Check sheet for the modelled part. Datum: model origin and axes. Units: mm. A direction names the side the tool comes from. Round coordinates to 2 decimals unless told otherwise and drop trailing zeros. Loops run counter-clockwise (first coordinate to the right, second up) from the corner with the lowest first, then second, coordinate; pieces in that order, holes last. Notation, with made-up numbers: (-21, 63.5) - (33, 63.5) arc R12 cw to (33, 86.5) - close; hole circle Ø8 at (-31.75, 0.25). An arc over 180 degrees is marked (long way). Put each result on its own line as item: value. Start each with the question number.
Item 1: Material ranges on line 1 along X through (y, z) = (-19.5, 0.5); line 2 along X through (y, z) = (-29.5, 0.5); line 3 along Y through (x, z) = (125.5, 4.5), recorded low to high.
Item 2: Gauge pin test, flat ends, axial feed: pin 1 Ø1.9 at (y, z) = (-72, 2) entering from +X; pin 2 Ø3 at (y, z) = (-93, 3) entering from -X; pin 3 Ø1.9 at (x, z) = (92.5, 2.5) entering from -Y; pin 4 Ø6.5 at (x, y) = (10.31, -38.66) entering from +Z. Record the tip position at first contact, or that the pin passes through.
Item 3: Section check C-C, the plane y = -54.5. Record the cut outline in (x, z).
Item 4: Section check A-A, the plane y = -30.5. Record the cut outline in (x, z).
Item 5: Section check B-B, the plane z = 3. Give the number of separate pieces and of enclosed holes in the cut face, and give its area (3 significant figures).
Item 6: Tool access check on faces 1 (the flat face through (85.725, -92, 3)), 2 (the flat face through (153, -38.1, 3)), 3 (the flat face through (-3, -19.05, 3)). Record the directions out of +Z, -Z, +X, -X, +Y, -Y that give a thin tool (end or side, any length) a straight path to the whole face; none if there is none.
Item 7: Draft check along X on faces 4 (the flat face through (156.21, -5, 3)), 5 (the flat face through (115.57, -19, 3)), 6 (the flat face through (133.35, -92, 3)), 7 (the flat face through (0, -14, 3)). Enter one of: pulls with the +X half, pulls with the -X half, needs draft (parallel to the pull), parting line crosses it, or undercut.
from build123d import *

# Parameters (mm, degrees)
SKETCH1_W           = 149.86
SKETCH1_H           = 88.9
SKETCH1_W_2         = 19.05
SKETCH1_H_2         = 6.35
GENERAL_SHAPE_DEPTH = 6.35
SKETCH4_R           = 2.0193
SLOT_CUT_OUTS_DEPTH = 6.35
SKETCH5_W           = 6.35
SKETCH5_H           = 9.525
SKETCH5_W_2         = 9.525
SKETCH5_H_2         = 6.35
EDGE_TEETH_DEPTH    = 6.35


with BuildPart() as part:
    # Sketch1 → General Shape (new body)
    with BuildSketch(Plane.XY):
        with Locations((74.93, -44.45)):
            Rectangle(SKETCH1_W, SKETCH1_H)
        with Locations((133.985, -79.375)):
            Rectangle(SKETCH1_W_2, SKETCH1_H_2, mode=Mode.SUBTRACT)
        with Locations((15.875, -79.375)):
            Rectangle(SKETCH1_W_2, SKETCH1_H_2, mode=Mode.SUBTRACT)
    extrude(amount=GENERAL_SHAPE_DEPTH)

    # Sketch4 → Slot Cut-Outs (cut)
    with BuildSketch(Plane.XY.offset(6.35)):
        with Locations((37.9476, -9.6266)):
            Circle(SKETCH4_R)
        with Locations((37.9476, -38.6588)):
            Circle(SKETCH4_R)
        with Locations((10.3124, -38.6588)):
            Circle(SKETCH4_R)
        with Locations((10.3124, -9.6266)):
            Circle(SKETCH4_R)
        with Locations((139.5476, -9.6266)):
            Circle(SKETCH4_R)
        with Locations((111.9124, -9.6266)):
            Circle(SKETCH4_R)
        with Locations((111.9124, -38.6588)):
            Circle(SKETCH4_R)
        with Locations((139.5476, -38.6588)):
            Circle(SKETCH4_R)
        with BuildLine():
            Line((34.29, 0), (34.29, -38.1))
            ThreePointArc((34.29, -38.1), (24.13, -48.26), (13.97, -38.1))
            Line((13.97, -38.1), (13.97, 0))
            ThreePointArc((13.97, 0), (24.13, 10.16), (34.29, 0))
        make_face()
        with BuildLine():
            Line((135.89, 0), (135.89, -38.1))
            ThreePointArc((135.89, -38.1), (125.73, -48.26), (115.57, -38.1))
            Line((115.57, -38.1), (115.57, 0))
            ThreePointArc((115.57, 0), (125.73, 10.16), (135.89, 0))
        make_face()
    extrude(amount=-SLOT_CUT_OUTS_DEPTH, mode=Mode.SUBTRACT)

    # Sketch5 → Edge Teeth (add)
    with BuildSketch(Plane.XY.offset(6.35)):
        with Locations((-3.175, -4.7625)):
            Rectangle(SKETCH5_W, SKETCH5_H)
        with Locations((-3.175, -23.8125)):
            Rectangle(SKETCH5_W, SKETCH5_H)
        with Locations((-3.175, -42.8625)):
            Rectangle(SKETCH5_W, SKETCH5_H)
        with Locations((-3.175, -61.9125)):
            Rectangle(SKETCH5_W, SKETCH5_H)
        with Locations((-3.175, -80.9625)):
            Rectangle(SKETCH5_W, SKETCH5_H)
        with Locations((153.035, -80.9625)):
            Rectangle(SKETCH5_W, SKETCH5_H)
        with Locations((153.035, -61.9125)):
            Rectangle(SKETCH5_W, SKETCH5_H)
        with Locations((153.035, -42.8625)):
            Rectangle(SKETCH5_W, SKETCH5_H)
        with Locations((153.035, -23.8125)):
            Rectangle(SKETCH5_W, SKETCH5_H)
        with Locations((153.035, -4.7625)):
            Rectangle(SKETCH5_W, SKETCH5_H)
        with Locations((23.8125, -92.075)):
            Rectangle(SKETCH5_W_2, SKETCH5_H_2)
        with Locations((4.7625, -92.075)):
            Rectangle(SKETCH5_W_2, SKETCH5_H_2)
        with Locations((42.8625, -92.075)):
            Rectangle(SKETCH5_W_2, SKETCH5_H_2)
        with Locations((61.9125, -92.075)):
            Rectangle(SKETCH5_W_2, SKETCH5_H_2)
        with Locations((80.9625, -92.075)):
            Rectangle(SKETCH5_W_2, SKETCH5_H_2)
        with Locations((100.0125, -92.075)):
            Rectangle(SKETCH5_W_2, SKETCH5_H_2)
        with Locations((119.0625, -92.075)):
            Rectangle(SKETCH5_W_2, SKETCH5_H_2)
        with Locations((138.1125, -92.075)):
            Rectangle(SKETCH5_W_2, SKETCH5_H_2)
    extrude(amount=-EDGE_TEETH_DEPTH)


solid = part.part
Check result:
1. line 1: -6.35 to 13.97, 34.29 to 115.57, 135.89 to 156.21
1. line 2: 0 to 13.97, 34.29 to 115.57, 135.89 to 149.86
1. line 3: -88.9 to -82.55, -76.2 to -48.26
2. pin 1: x = 149.86
2. pin 2: x = 0
2. pin 3: y = -88.9
2. pin 4: z = 6.35
3. outline: (0, 0) - (149.86, 0) - (149.86, 6.35) - (0, 6.35) - close
4. outline: (0, 0) - (13.97, 0) - (13.97, 6.35) - (0, 6.35) - close; (34.29, 0) - (115.57, 0) - (115.57, 6.35) - (34.29, 6.35) - close; (135.89, 0) - (149.86, 0) - (149.86, 6.35) - (135.89, 6.35) - close
5. separate pieces: 1
5. enclosed holes: 10
5. area: 12,200 mm²
6. face 1: +Z, -Z, -Y
6. face 2: +Z, -Z, +X
6. face 3: +Z, -Z, -X
7. face 4: pulls with the +X half
7. face 5: undercut
7. face 6: undercut
7. face 7: pulls with the -X half
